CAD build for the part. Positions are in the model's coordinates, mm. A direction names the side the tool comes from. Coordinates: 2 decimals unless noted, no trailing zeros. Order: outer loops, then holes, each group sorted by start corner. A loop starts at its lowest first (then second) coordinate and runs counter-clockwise, first axis right, second up. Notation, with made-up numbers: (-24, 6.25) - (18, 6.25) arc R11 cw to (18, 15.25) - close; hole circle Ø2 at (-5.5, 6.25). An arc over 180 degrees is marked (long way). Use one line per item in the form item = value.
```python
from build123d import *

# Parameters (mm, degrees)
ESQUISSE1_W             = 16
ESQUISSE1_H             = 30
ESQUISSE1_R             = 1.75
BOSS_EXTRU_1_DEPTH      = 8
ESQUISSE2_R             = 5.15
ENL_V_MAT_EXTRU_1_DEPTH = 5
CONG_1_R                = 5
ENL_V_MAT_EXTRU_2_DEPTH = 4
CONG_2_R                = 3


with BuildPart() as part:
    # Esquisse1 → Boss.-Extru.1 (new body)
    with BuildSketch(Plane(origin=(0, 0, 0), x_dir=(1, 0, 0), z_dir=(0, 1, 0))):
        with Locations((8, 15)):
            Rectangle(ESQUISSE1_W, ESQUISSE1_H)
        with Locations(Location((8, 25, 0), (0, 0, 270))):
            Circle(ESQUISSE1_R, mode=Mode.SUBTRACT)
        with Locations(Location((8, 5, 0), (0, 0, 90))):
            Circle(ESQUISSE1_R, mode=Mode.SUBTRACT)
    extrude(amount=BOSS_EXTRU_1_DEPTH)

    # Esquisse2 → Enlèv. mat.-Extru.1 (cut)
    with BuildSketch(Plane(origin=(0, 8, 0), x_dir=(1, 0, 0), z_dir=(0, 1, 0))):
        with Locations(Location((8, 15, 0), (0, 0, 270))):
            Circle(ESQUISSE2_R)
    extrude(amount=-ENL_V_MAT_EXTRU_1_DEPTH, mode=Mode.SUBTRACT)

    # Congé1
    cong_1_edges = [part.edges().sort_by_distance(p)[0] for p in [
        (0, 4, -30),
        (16, 4, -30),
        (16, 4, 0),
        (0, 4, 0),
    ]]
    fillet(cong_1_edges, radius=CONG_1_R)

    # Esquisse3 → Enlèv. mat.-Extru.2 (cut)
    with BuildSketch(Plane(origin=(0, 8, 0), x_dir=(1, 0, 0), z_dir=(0, 1, 0))):
        Polygon((6.354551733, 27.85), (9.645448267, 27.85), (11.290896534, 25), (9.645448267, 22.15), (6.354551733, 22.15), (4.709103466, 25), align=None)
        Polygon((6.354551733, 7.85), (9.645448267, 7.85), (11.290896534, 5), (9.645448267, 2.15), (6.354551733, 2.15), (4.709103466, 5), align=None)
    extrude(amount=-ENL_V_MAT_EXTRU_2_DEPTH, mode=Mode.SUBTRACT)

    # Congé2
    # the kernel refuses this fillet: 3 mm, written as the material it takes off along each edge
    with BuildSketch(Plane(origin=(5, 8, -5), x_dir=(0, 0, 1), z_dir=(1, 0, 0))) as cong_2_piece_1:
        with BuildLine():
            CenterArc((5 - CONG_2_R, CONG_2_R), CONG_2_R, 270, 90)
            Line((5 - CONG_2_R, 0), (5, 0))
            Line((5, 0), (5, CONG_2_R))
        make_face()
    revolve(axis=Axis((5, 8, -5), (0, -1, 0)), revolution_arc=90, mode=Mode.SUBTRACT)
    with BuildSketch(Plane(origin=(0, 8, -25), x_dir=(1, 0, 0), z_dir=(0, 0, 1)), Plane(origin=(16, 8, -5), x_dir=(-1, 0, 0), z_dir=(0, 0, -1))) as cong_2_piece_2:
        with BuildLine():
            CenterArc((CONG_2_R, -CONG_2_R), CONG_2_R, 90, 90)
            Line((0, -CONG_2_R), (0, 0))
            Line((0, 0), (CONG_2_R, 0))
        make_face()
    extrude(amount=20, mode=Mode.SUBTRACT)
    with BuildSketch(Plane(origin=(5, 8, -25), x_dir=(-1, 0, 0), z_dir=(0, 0, 1))) as cong_2_piece_3:
        with BuildLine():
            CenterArc((5 - CONG_2_R, CONG_2_R), CONG_2_R, 270, 90)
            Line((5, CONG_2_R), (5, 0))
            Line((5, 0), (5 - CONG_2_R, 0))
        make_face()
    revolve(axis=Axis((5, 8, -25), (0, -1, 0)), revolution_arc=90, mode=Mode.SUBTRACT)
    with BuildSketch(Plane(origin=(11, 8, -30), x_dir=(0, 0, 1), z_dir=(-1, 0, 0))) as cong_2_piece_4:
        with BuildLine():
            CenterArc((CONG_2_R, -CONG_2_R), CONG_2_R, 90, 90)
            Line((0, -CONG_2_R), (0, 0))
            Line((0, 0), (CONG_2_R, 0))
        make_face()
    extrude(amount=6, mode=Mode.SUBTRACT)
    with BuildSketch(Plane(origin=(11, 8, -25), x_dir=(1, 0, 0), z_dir=(0, 0, 1))) as cong_2_piece_5:
        with BuildLine():
            CenterArc((5 - CONG_2_R, -CONG_2_R), CONG_2_R, 0, 90)
            Line((5, -CONG_2_R), (5, 0))
            Line((5, 0), (5 - CONG_2_R, 0))
        make_face()
    revolve(axis=Axis((11, 8, -25), (0, 1, 0)), revolution_arc=90, mode=Mode.SUBTRACT)
    with BuildSketch(Plane(origin=(11, 8, -5), x_dir=(0, 0, 1), z_dir=(-1, 0, 0))) as cong_2_piece_6:
        with BuildLine():
            CenterArc((5 - CONG_2_R, -CONG_2_R), CONG_2_R, 0, 90)
            Line((5 - CONG_2_R, 0), (5, 0))
            Line((5, 0), (5, -CONG_2_R))
        make_face()
    revolve(axis=Axis((11, 8, -5), (0, 1, 0)), revolution_arc=90, mode=Mode.SUBTRACT)
    with BuildSketch(Plane(origin=(5, 8, 0), x_dir=(0, -1, 0), z_dir=(1, 0, 0))) as cong_2_piece_7:
        with BuildLine():
            CenterArc((CONG_2_R, CONG_2_R), CONG_2_R, 180, 90)
            Line((0, CONG_2_R), (0, 0))
            Line((0, 0), (CONG_2_R, 0))
        make_face()
    extrude(amount=6, mode=Mode.SUBTRACT)


solid = part.part
```
Item 1: Cut at A-A, the plane y = 3.5. Write the cut outline in (x, z), plus the area to 3 significant figures.
Derived:
outline = (0, -25) arc R5 ccw to (5, -30) - (11, -30) arc R5 ccw to (16, -25) - (16, -5) arc R5 ccw to (11, 0) - (5, 0) arc R5 ccw to (0, -5) - close; hole circle Ø10.3 at (8, -15); hole circle Ø3.5 at (8, -25); hole circle Ø3.5 at (8, -5)
area = 356 mm²
Item 2: 3-axis set-ups, long thin cutter, end or side, ignore diameter. For faces 5 (the face through (7.958, 6.748, -0.562)), 6 (the face through (10.46, 6.03, -26.44)): which of +Z, -Z, +X, -X, +Y, -Y reach the whole face in a straight line?
Derived:
face_5 = +Z, +X, -X, +Y
face_6 = +Y
Item 3: Cut at B-B, the plane y = 2.25. Write the cut outline in (x, z), plus the area to 3 significant figures.
Derived:
outline = (0, -25) arc R5 ccw to (5, -30) - (11, -30) arc R5 ccw to (16, -25) - (16, -5) arc R5 ccw to (11, 0) - (5, 0) arc R5 ccw to (0, -5) - close; hole circle Ø3.5 at (8, -25); hole circle Ø3.5 at (8, -5)
area = 439 mm²
Item 4: Cut at C-C, the plane x = 8. Write the cut outline in (y, z).
Derived:
outline = (0, -30) - (5, -30) arc R3 ccw to (7.88, -27.85) - (4, -27.85) - (4, -26.75) - (0, -26.75) - close; (0, -23.25) - (4, -23.25) - (4, -22.15) - (8, -22.15) - (8, -20.15) - (3, -20.15) - (3, -9.85) - (8, -9.85) - (8, -7.85) - (4, -7.85) - (4, -6.75) - (0, -6.75) - close; (0, -3.25) - (4, -3.25) - (4, -2.15) - (7.88, -2.15) arc R3 ccw to (5, 0) - (0, 0) - close
Item 5: Drop flat-ended pins along their axis: pin 1 (3 mm diameter, centred on y = 6, z = -6.5, fed in from -X); pin 2 (3 mm diameter, centred on x = 5.5, z = -15.5, fed in from +Y); pin 3 (3 mm diameter, centred on x = 8, z = -5, fed in from +Y); pin 4 (1 mm diameter, centred on x = 3, y = 3.5, fed in from +Z). Give the stop position or say it passes through.
Derived:
pin_1 = 0
pin_2 = 3
pin_3 = through
pin_4 = -0.23
Item 6: Drill centre lines: line 1 (Z direction, x = 8, y = 1.3); line 2 (X direction, y = 1.35, z = -25); line 3 (Z direction, x = 8, y = 5.3). Where is each one in solid material? Low to high. Write a range as [from, to].
Derived:
line_1 = [-30, -26.75], [-23.25, -6.75], [-3.25, 0]
line_2 = [0, 6.25], [9.75, 16]
line_3 = [-29.98, -27.85], [-22.15, -20.15], [-9.85, -7.85], [-2.15, -0.02]
Item 7: Cut at D-D, the plane z = -7.25. Write the cut outline in (x, y), plus the area to 3 significant figures.
Derived:
outline = (0, 0) - (16, 0) - (16, 5) arc R3 ccw to (13, 8) - (9.99, 8) - (9.99, 4) - (6.01, 4) - (6.01, 8) - (3, 8) arc R3 ccw to (0, 5) - close
area = 108 mm²
Item 8: Two-plate mould, pull along X, no slides. Class faces 1 (the face through (10.48, 6.028, -23.595)), 2 (the face through (0, 2, -15)), 3 (the face through (16, 2, -15)), 4 (the face through (8.08, 1.97, -26.75)): +X half, -X half, draft (parallel to the pull), parting line (faces both ways), or undercut.
Derived:
face_1 = undercut
face_2 = -X half
face_3 = +X half
face_4 = undercut
